Work out the finished part from the listing and answer in its coordinate system (mm). Round coordinates to 2 decimals unless told otherwise and drop trailing zeros. Write each loop counter-clockwise with the first axis right and the second up, starting at its lowest first coordinate (ties: lowest second). Pieces come first, ordered by that corner, then holes. Notation, with made-up numbers: M -29.5,-28.75 L -16.5,-28.75 A26 ccw -16.5,-4.75 Z; hole C 59,31.5 d1. An arc over 180 degrees is marked long. One line per item, written item: value. Start each with the question number.
Q1. Find section C-C (x = -16.5). Write down the section's boundary in (y, z).
Q2. Find section B-B (z = 6). Count the separate pieces of the cut face and the enclosed holes in it, and give its area (3 significant figures).
Q3. Given pin 1 Ø3 at (x, y) = (-43.95, -9.33) entering from +Z, flat-ended and moving along its own axis, determine where the tip first touches the part or whether it passes through.
Q4. Find section A-A (y = 0). Write down the section's boundary in (x, z), and give its area (3 significant figures).
Q5. Consider probe 1 along Y at (x, z) = (-16, 5); probe 2 along Y at (x, z) = (-43, 6); probe 3 along Z at (x, y) = (-43.5, -0.75). Determine where each line is inside the solid, lowest interval first.
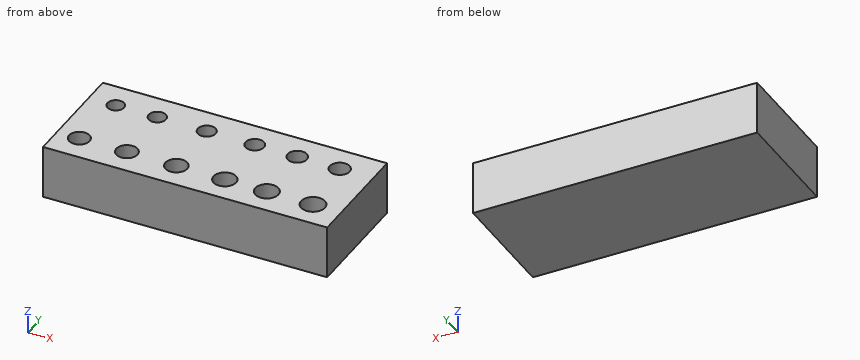
from build123d import *

# Parameters (mm, degrees)
F0_W     = 42.807285
F0_H     = 17.540547
F0_R     = 1.55
F0_R_2   = 1.6
F0_R_3   = 1.65
F0_R_4   = 1.7
F0_R_5   = 1.75
F0_R_6   = 1.8
F0_R_7   = 1.25
F0_R_8   = 1.3
F0_R_9   = 1.35
F0_R_10  = 1.4
F0_R_11  = 1.45
F0_R_12  = 1.5
F1_DEPTH = 8
F2_DEPTH = 2


with BuildPart() as f1:
    # F0 (on Top) → F1 (new body)
    with BuildSketch(Plane.XY):
        with Locations((-25.905089, -4.67933)):
            Rectangle(F0_W, F0_H)
        with Locations((-43.950986, -9.325703)):
            Circle(F0_R, mode=Mode.SUBTRACT)
        with Locations((-36.78672, -9.325703)):
            Circle(F0_R_2, mode=Mode.SUBTRACT)
        with Locations((-29.344233, -9.325703)):
            Circle(F0_R_3, mode=Mode.SUBTRACT)
        with Locations((-22.040857, -9.325703)):
            Circle(F0_R_4, mode=Mode.SUBTRACT)
        with Locations((-15.711265, -9.325703)):
            Circle(F0_R_5, mode=Mode.SUBTRACT)
        with Locations((-8.755669, -9.325703)):
            Circle(F0_R_6, mode=Mode.SUBTRACT)
        with Locations((-43.255426, 0)):
            Circle(F0_R_7, mode=Mode.SUBTRACT)
        with Locations((-36.995389, 0)):
            Circle(F0_R_8, mode=Mode.SUBTRACT)
        with Locations((-29.552901, 0)):
            Circle(F0_R_9, mode=Mode.SUBTRACT)
        with Locations((-22.319082, 0)):
            Circle(F0_R_10, mode=Mode.SUBTRACT)
        with Locations((-15.919933, 0)):
            Circle(F0_R_11, mode=Mode.SUBTRACT)
        with Locations((-9.520785, 0)):
            Circle(F0_R_12, mode=Mode.SUBTRACT)
    extrude(amount=F1_DEPTH)

    # F0 (on Top) → F2 (join)
    with BuildSketch(Plane.XY):
        with Locations((-43.950986, -9.325703)):
            Circle(F0_R)
        with Locations((-36.78672, -9.325703)):
            Circle(F0_R_2)
        with Locations((-29.344233, -9.325703)):
            Circle(F0_R_3)
        with Locations((-22.040857, -9.325703)):
            Circle(F0_R_4)
        with Locations((-15.711265, -9.325703)):
            Circle(F0_R_5)
        with Locations((-8.755669, -9.325703)):
            Circle(F0_R_6)
        with Locations((-9.520785, 0)):
            Circle(F0_R_12)
        with Locations((-15.919933, 0)):
            Circle(F0_R_11)
        with Locations((-22.319082, 0)):
            Circle(F0_R_10)
        with Locations((-29.552901, 0)):
            Circle(F0_R_9)
        with Locations((-36.995389, 0)):
            Circle(F0_R_8)
        with Locations((-43.255426, 0)):
            Circle(F0_R_7)
    extrude(amount=F2_DEPTH)


solid = f1.part
The answers:
1. outline: M -13.45,0 L 4.09,0 L 4.09,8 L 1.33,8 L 1.33,2 L -1.33,2 L -1.33,8 L -7.76,8 L -7.76,2 L -10.89,2 L -10.89,8 L -13.45,8 Z
2. separate pieces: 1
2. enclosed holes: 12
2. area: 662 mm2
3. pin 1: z = 2
4. outline: M -47.31,0 L -4.5,0 L -4.5,8 L -8.02,8 L -8.02,2 L -11.02,2 L -11.02,8 L -14.47,8 L -14.47,2 L -17.37,2 L -17.37,8 L -20.92,8 L -20.92,2 L -23.72,2 L -23.72,8 L -28.2,8 L -28.2,2 L -30.9,2 L -30.9,8 L -35.7,8 L -35.7,2 L -38.3,2 L -38.3,8 L -42.01,8 L -42.01,2 L -44.51,2 L -44.51,8 L -47.31,8 Z
4. area: 243 mm2
5. probe 1: -13.45 to -11.05, -7.6 to -1.45, 1.45 to 4.09
5. probe 2: -13.45 to -10.55, -8.1 to -1.22, 1.22 to 4.09
5. probe 3: 0 to 2
